Read the model definition and answer for the solid it produces. Units are mm, in the model's axes. Coordinates: 2 decimals unless noted, no trailing zeros. Loops run counter-clockwise (first coordinate to the right, second up) from the corner with the lowest first, then second, coordinate; pieces in that order, holes last.
from build123d import *

# Parameters (mm, degrees)
SKETCH1_R           = 12.7
SKETCH1_R_2         = 5
SKETCH1_R_3         = 1.27
BOSS_EXTRUDE1_DEPTH = 3.175
FILLET1_R           = 2.54
FILLET2_R           = 2.54


with BuildPart() as part:
    # Sketch1 → Boss-Extrude1 (new body)
    with BuildSketch(Plane(origin=(0, 0, 0), x_dir=(0, 0, -1), z_dir=(1, 0, 0))):
        with BuildLine():
            Line((-19.05, -16.938), (0, -16.938))
            Line((0, -16.938), (19.05, -16.938))
            Line((19.05, -16.938), (12.045339341, 4.024897535))
            ThreePointArc((12.045339341, 4.024897535), (12.535266444, 2.03889558), (12.7, 0))
            ThreePointArc((12.7, 0), (-2.03889558, -12.535266444), (-12.045339341, 4.024897535))
            Line((-12.045339341, 4.024897535), (-19.05, -16.938))
        make_face()
        Circle(SKETCH1_R)
        Circle(SKETCH1_R_2, mode=Mode.SUBTRACT)
        with Locations((-8.5, 0)):
            Circle(SKETCH1_R_3, mode=Mode.SUBTRACT)
        with Locations((8.5, 0)):
            Circle(SKETCH1_R_3, mode=Mode.SUBTRACT)
    extrude(amount=-BOSS_EXTRUDE1_DEPTH)

    # Fillet1
    fillet1_edges = [part.edges().sort_by_distance(p)[0] for p in [
        (-1.5875, -16.938, -19.05),
    ]]
    fillet(fillet1_edges, radius=FILLET1_R)

    # Fillet2
    fillet2_edges = [part.edges().sort_by_distance(p)[0] for p in [
        (-1.5875, -16.938, 19.05),
    ]]
    fillet(fillet2_edges, radius=FILLET2_R)


solid = part.part
Q1. A cutting plane is placed at A-A (x = -1.6). Give the vertices of the cut face in (y, z).
Findings below:
outline: (-16.94, -15.52) arc R2.54 ccw to (-13.59, -17.93) - (4.02, -12.05) arc R12.7 ccw to (4.02, 12.05) - (-13.59, 17.93) arc R2.54 ccw to (-16.94, 15.52) - close; hole circle Ø10 at (0, 0); hole circle Ø2.54 at (0, -8.5); hole circle Ø2.54 at (0, 8.5)
Q2. A cutting plane is placed at D-D (z = 0). Give the vertices of the cut face in (x, y) (3 decimals), then the cut area to 3 significant figures.
Findings below:
outline: (-3.175, -16.938) - (0, -16.938) - (0, -5) - (-3.175, -5) - close; (-3.175, 5) - (0, 5) - (0, 12.7) - (-3.175, 12.7) - close
area: 62.4 mm2
Q3. A flat-ended cylindrical pin translates along its axis: pin 1 Ø1.5 at (x, y) = (-2, 1) entering from +Z. Find the tip coordinate at first contact, or state that the pin passes through.
Findings below:
pin 1: stops at z = 13.31
Q4. A cutting plane is placed at B-B (y = 0). Give the vertices of the cut face in (x, z) (3 decimals), then the cut area to 3 significant figures.
Findings below:
outline: (-3.175, -13.39) - (0, -13.39) - (0, -9.77) - (-3.175, -9.77) - close; (-3.175, -7.23) - (0, -7.23) - (0, -5) - (-3.175, -5) - close; (-3.175, 5) - (0, 5) - (0, 7.23) - (-3.175, 7.23) - close; (-3.175, 9.77) - (0, 9.77) - (0, 13.39) - (-3.175, 13.39) - close
area: 37.1 mm2
Q5. Straight lines are drawn through the part: probe 1 along Y at (x, z) = (-2.45, 0); probe 2 along Y at (x, z) = (-1, -8.5); probe 3 along Z at (x, y) = (-2.1, -1.5). For each, find the intervals that lie inside material, in ascending order.
Findings below:
probe 1: y = -16.94 to -5, 5 to 12.7
probe 2: y = -16.94 to -1.27, 1.27 to 9.44
probe 3: z = -13.89 to -4.77, 4.77 to 13.89
Q6. Determine the mould class of faces 1 (the face through (-1.57, -0.49, -9.67)), 2 (the face through (-1.57, -4.91, -15.03)), 3 (the face through (-1.61, -15.91, -17.564)) for opening direction Y: +Y half, -Y half, draft (parallel to the pull), parting line (faces both ways), or undercut.
Findings below:
face 1: undercut
face 2: +Y half
face 3: parting line
Q7. A cutting plane is placed at C-C (z = 8.5). Give the vertices of the cut face in (x, y) (3 decimals).
Findings below:
outline: (-3.175, -16.938) - (0, -16.938) - (0, -1.27) - (-3.175, -1.27) - close; (-3.175, 1.27) - (0, 1.27) - (0, 9.436) - (-3.175, 9.436) - close
